Geometry check sheet. Reference: the model listing, model coordinates, mm. A direction names the side the tool comes from. Give positions to 0.01 mm unless a question says otherwise; leave off trailing zeros. Write each loop counter-clockwise with the first axis right and the second up, starting at its lowest first coordinate (ties: lowest second). Pieces come first, ordered by that corner, then holes. Notation, with made-up numbers: (36.5, -16) -> (86.5, -16) arc R14 ccw to (86.5, -3) -> close; hole circle Ø6 at (-31, -21). An arc over 180 degrees is marked (long way). Use a Markdown table: item, result. Add a question column.
from build123d import *

# Parameters (mm, degrees)
F0_W     = 50.8
F0_H     = 50.8
F1_DEPTH = 50.8
F2_W     = 44.45
F2_H     = 44.66816
F3_DEPTH = 48.26
F4_R     = 36.802798
F5_DEPTH = 50.8
F7_DEPTH = 48.26


with BuildPart() as f1:
    # F0 (on Top) → F1 (new body)
    with BuildSketch(Plane.XY):
        Rectangle(F0_W, F0_H)
    extrude(amount=F1_DEPTH)

    # F2 (on face) → F3 (cut)
    with BuildSketch(Plane.XY.offset(50.8)):
        Rectangle(F2_W, F2_H)
    extrude(amount=-F3_DEPTH, mode=Mode.SUBTRACT)

    # F4 (on Top) → F5 (join)
    with BuildSketch(Plane.XY):
        Circle(F4_R)
    extrude(amount=F5_DEPTH)

    # F2 (on face) → F7 (cut)
    with BuildSketch(Plane.XY.offset(50.8)):
        Rectangle(F2_W, F2_H)
    extrude(amount=-F7_DEPTH, mode=Mode.SUBTRACT)


solid = f1.part
1) Sectioned sample at D-D, the plane x = -23.5. Enter the section's corners in (y, z), and give its area (3 significant figures).
2) Gauge pin test, flat ends, axial feed: P1, Ø5, axis at x = -22, z = 5, coming from the -Y side; P2, Ø3, axis at x = 27.5, y = 23, coming from the -Z side; P3, Ø22, axis at x = -9.5, z = 33, coming from the -Y side; P4, Ø5, axis at y = -22.5, z = 24, coming from the -X side. Record the tip position at first contact, or that the pin passes through.
3) Sectioned sample at B-B, the plane y = 0. Enter the section's corners in (x, z) (3 decimals), and give its area (3 significant figures).
4) Sectioned sample at A-A, the plane z = 37.5. Enter the section's corners in (x, y) (3 decimals).
5) Draft check along Y on faces 1 (the face through (0, 22.334, 27)), 2 (the face through (0, 0, 2.54)), 3 (the face through (-1, -24, 50.8)), 4 (the face through (16.98, -32.65, 25.04)). Enter one of: +Y half, -Y half, draft (parallel to the pull), parting line (faces both ways), or undercut.
6) Tool access check on faces 5 (the face through (-22.225, 0, 27)), 6 (the face through (-1, 1, 0)). Record the directions out of +Z, -Z, +X, -X, +Y, -Y that give a thin tool (end or side, any length) a straight path to the whole face; none if there is none.
7) Material ranges on probe 1 along X at (y, z) = (1, 29) (3 decimals); probe 2 along Y at (x, z) = (0.5, 25); probe 3 along Z at (x, y) = (12, -22), recorded low to high. Write a range as [from, to].
8) Sectioned sample at C-C, the plane x = 0. Enter the section's corners in (y, z).
Check values:
| question | item | result |
|---|---|---|
| 1 | outline | (-28.32, 0) -> (28.32, 0) -> (28.32, 50.8) -> (-28.32, 50.8) -> close |
| 1 | area | 2,880 mm² |
| 2 | P1 | y = -31.21 |
| 2 | P2 | z = 0 |
| 2 | P3 | y = -36.8 |
| 2 | P4 | x = -30.89 |
| 3 | outline | (-36.803, 0) -> (36.803, 0) -> (36.803, 50.8) -> (22.225, 50.8) -> (22.225, 2.54) -> (-22.225, 2.54) -> (-22.225, 50.8) -> (-36.803, 50.8) -> close |
| 3 | area | 1,590 mm² |
| 4 | outline | circle Ø73.606 at (0, 0); hole (-22.225, -22.334) -> (22.225, -22.334) -> (22.225, 22.334) -> (-22.225, 22.334) -> close |
| 5 | face 1 | undercut |
| 5 | face 2 | undercut |
| 5 | face 3 | draft |
| 5 | face 4 | parting line |
| 6 | face 5 | +Z |
| 6 | face 6 | -Z, +X, -X, +Y, -Y |
| 7 | probe 1 | [-36.789, -22.225], [22.225, 36.789] |
| 7 | probe 2 | [-36.8, -22.33], [22.33, 36.8] |
| 7 | probe 3 | [0, 2.54] |
| 8 | outline | (-36.8, 0) -> (36.8, 0) -> (36.8, 50.8) -> (22.33, 50.8) -> (22.33, 2.54) -> (-22.33, 2.54) -> (-22.33, 50.8) -> (-36.8, 50.8) -> close |
